from build123d import *

# Parameters (mm, degrees)
F0_W     = 25.4
F0_H     = 25.4
F1_DEPTH = 279.4
F2_W     = 149.225
F2_H     = 6.35
F3_DEPTH = 25.4


with BuildPart() as f1:
    # F0 (on Front) → F1 (new body)
    with BuildSketch(Plane.XZ):
        with Locations((12.7, 12.7)):
            Rectangle(F0_W, F0_H)
    extrude(amount=F1_DEPTH)

    # F2 (on face) → F3 (cut)
    with BuildSketch(Plane.YZ.offset(25.4)):
        with BuildLine():
            ThreePointArc((-263.525, 12.7), (-266.7, 15.875), (-269.875, 12.7))
            Line((-269.875, 12.7), (-266.7, 12.7))
            Line((-266.7, 12.7), (-266.7, 9.525))
            ThreePointArc((-266.7, 9.525), (-264.454936, 10.454936), (-263.525, 12.7))
        make_face()
        with BuildLine():
            Line((-266.7, 12.7), (-269.875, 12.7))
            ThreePointArc((-269.875, 12.7), (-268.945064, 10.454936), (-266.7, 9.525))
            Line((-266.7, 9.525), (-266.7, 12.7))
        make_face()
        with BuildLine():
            ThreePointArc((-184.15, 15.875), (-187.325, 12.7), (-184.15, 9.525))
            Line((-184.15, 9.525), (-184.15, 15.875))
        make_face()
        with Locations((-109.5375, 12.7)):
            Rectangle(F2_W, F2_H)
        with BuildLine():
            ThreePointArc((-34.925, 9.525), (-32.679936, 10.454936), (-31.75, 12.7))
            ThreePointArc((-31.75, 12.7), (-32.679936, 14.945064), (-34.925, 15.875))
            Line((-34.925, 15.875), (-34.925, 9.525))
        make_face()
    extrude(amount=-F3_DEPTH, mode=Mode.SUBTRACT)


solid = f1.part
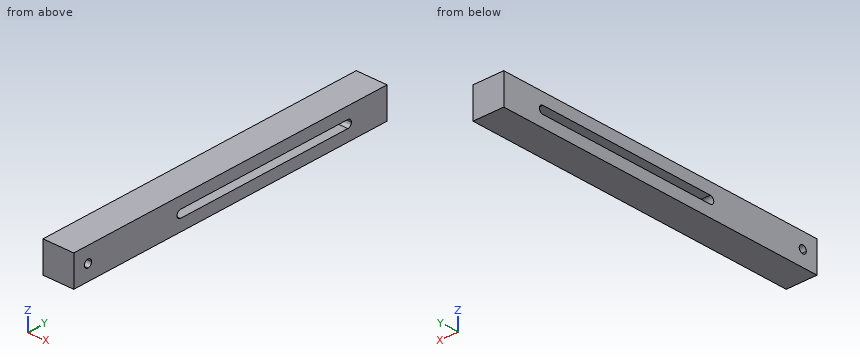
For this review, take the finished solid that the model builds, in its own axes (mm). Round coordinates to 2 decimals unless told otherwise and drop trailing zeros. Write each loop counter-clockwise with the first axis right and the second up, starting at its lowest first coordinate (ties: lowest second). Pieces come first, ordered by that corner, then holes. Notation, with made-up numbers: (79, -10) -> (98, -10) arc R26 ccw to (98, 24) -> close; hole circle Ø2 at (12.5, 43.25). An arc over 180 degrees is marked (long way). Put each result on its own line as item: value.
Q1. To check wall thickness, follow L1, parallel to Y at x = 21, z = 12.25; L2, parallel to Z at x = 22.25, y = -97 (3 decimals); L3, parallel to Y at x = 14, z = 14.25. State the ranges of each line that lie inside material, in increasing order. Write a range as [from, to].
Determined:
L1: y = [-279.4, -269.84], [-263.56, -187.29], [-31.78, 0]
L2: z = [0, 9.525], [15.875, 25.4]
L3: y = [-279.4, -269.47], [-263.93, -186.92], [-32.15, 0]
Q2. Consider section A-A on y = -54.5. State the section outline as (x, z) points (3 decimals), and give its area (3 significant figures).
Determined:
outline: (0, 0) -> (25.4, 0) -> (25.4, 9.525) -> (0, 9.525) -> close; (0, 15.875) -> (25.4, 15.875) -> (25.4, 25.4) -> (0, 25.4) -> close
area: 484 mm^2
Q3. Consider section B-B on x = 15. State the section outline as (y, z) points (3 decimals), and give its area (3 significant figures).
Determined:
outline: (-279.4, 0) -> (0, 0) -> (0, 25.4) -> (-279.4, 25.4) -> close; hole circle Ø6.35 at (-266.7, 12.7); hole (-184.15, 9.525) -> (-34.925, 9.525) arc R3.175 ccw to (-34.925, 15.875) -> (-184.15, 15.875) arc R3.175 ccw to start
area: 6,090 mm^2
